Work out the finished part from the listing and answer in its coordinate system (mm). A direction names the side the tool comes from. Give positions to 0.01 mm unless a question says otherwise; leave off trailing zeros. Order: outer loops, then holes, each group sorted by start corner. A loop starts at its lowest first (then second) coordinate and runs counter-clockwise, first axis right, second up.
Autodesk Inventor part; units mm, degrees
ref_plane "YZ Plane" through (0, 0, 0) normal (1, 0, 0) x (0, 1, 0)
ref_plane "XZ Plane" through (0, 0, 0) normal (0, 1, 0) x (-1, 0, 0)
ref_plane "XY Plane" through (0, 0, 0) normal (0, 0, 1) x (1, 0, 0)
sketch "Sketch9" plane through (0, 0, 0) normal (0, 1, 0) x (-1, 0, 0)
  line L0 (-27, 35.5) -> (27, 35.5)
  line L1 (27, 35.5) -> (27, -35.5)
  line L2 (27, -35.5) -> (-27, -35.5)
  line L3 (-27, -35.5) -> (-27, 35.5)
  line L4 (-27, 35.5) -> (27, -35.5) construction
  line L5 (27, 35.5) -> (-27, -35.5) construction
  point P0 (0, 0)
  dimension "d39" = 54
  dimension "d40" = 71
extrude "Extrusion4" add sketch "Sketch9" along normal blind 10
sketch "Sketch10" plane through (0, 10, 0) normal (0, 1, 0) x (1, 0, 0)
  circle A0 centre (0, 0) radius 7.5
  dimension "d43" = 15
extrude "Extrusion5" cut sketch "Sketch10" against normal blind 10
sketch "Sketch11" plane through (27, 0, 35.5) normal (1, 0, 0) x (0, 0, -1)
  point P0 (35.5, 0)
  point P1 (35.5, 5)
hole "Hole5" at (27, 5, 0) direction (-1, 0, 0) diameter 3.242 depth 11.8 tip angle 118
sketch "Sketch12" plane through (0, 10, 0) normal (0, 1, 0) x (1, 0, 0)
  point P0 (0, 0)
sketch "Sketch13" plane through (0, 10, 0) normal (0, 1, 0) x (1, 0, 0)
  point P0 (0, 0)
  point P1 (22.809, -31.309)
  point P2 (-22.809, 31.309)
  point P3 (-22.809, -31.309)
  point P4 (22.809, 31.309)
hole "Hole6" at (-22.809, 10, 31.309) at (-22.809, 10, -31.309) at (22.809, 10, -31.309) at (22.809, 10, 31.309) direction (0, -1, 0) diameter 2.459 depth 8.8 tip angle 118
fillet "Fillet3" radius 4 4 edges at (-27, 5, -35.5) (-27, 5, 35.5) (27, 5, -35.5) (27, 5, 35.5)
sketch "Sketch14" plane through (23, 0, -35.5) normal (0, 0, -1) x (-1, 0, 0)
  point P0 (23, 0)
  point P1 (23, 5)
sketch "Sketch15" plane through (-23, 0, 35.5) normal (0, 0, 1) x (1, 0, 0)
  point P0 (23, 0)
  point P1 (23, 5)
hole "Hole7" at (0, 5, 35.5) direction (0, 0, -1) diameter 4 depth 20
hole "Hole8" at (0, 5, -35.5) direction (0, 0, 1) diameter 4 depth 20
sketch "Sketch16" plane through (0, 5, 15.5) normal (0, 0, 1) x (1, 0, 0)
  point P0 (0, -5)
  point P1 (0, 0)
sketch "Sketch17" plane through (0, 5, -15.5) normal (0, 0, -1) x (-1, 0, 0)
  point P0 (0, -5)
  point P1 (0, 0)
hole "Hole9" at (0, 5, -15.5) direction (0, 0, 1) diameter 3.242 depth 11.8
hole "Hole10" at (0, 5, 15.5) direction (0, 0, -1) diameter 3.242 depth 11.8
equation "\"z\" = 71"
equation "\"x\" = 54"
equation "\"corner\" = 4"
properties part number "CardMount_sjc"
1. The mould has two halves that part along X. Classify faces 1 (the face through (27, 3, 0)), 2 (the face through (-0.3, 2.7, -35.5)), 3 (the face through (1.2, 6.6, 25.4)): pulls with the +X half, pulls with the -X half, needs draft (parallel to the pull), parting line crosses it, or undercut.
Findings below:
face 1: pulls with the +X half
face 2: needs draft
face 3: undercut
2. The part is cut by section C-C (y = 8.5). Write down the section's boundary in (x, z), then the cut area to 3 significant figures.
Findings below:
outline: (-27, -31.5) arc R4 ccw to (-23, -35.5) - (23, -35.5) arc R4 ccw to (27, -31.5) - (27, 31.5) arc R4 ccw to (23, 35.5) - (-23, 35.5) arc R4 ccw to (-27, 31.5) - close; hole circle Ø2.46 at (-22.81, -31.31); hole circle Ø2.46 at (-22.81, 31.31); hole circle Ø15 at (0, 0); hole circle Ø2.46 at (22.81, -31.31); hole circle Ø2.46 at (22.81, 31.31)
area: 3,620 mm2
3. The part is cut by section B-B (z = -25.5). Write down the section's boundary in (x, y), then the cut area to 3 significant figures.
Findings below:
outline: (-27, 0) - (27, 0) - (27, 10) - (-27, 10) - close; hole circle Ø4 at (0, 5)
area: 527 mm2
4. The part is cut by section A-A (x = 0). Write down the section's boundary in (y, z).
Findings below:
outline: (0, -35.5) - (3, -35.5) - (3, -15.5) - (3.38, -15.5) - (3.38, -7.5) - (0, -7.5) - close; (0, 7.5) - (3.38, 7.5) - (3.38, 15.5) - (3, 15.5) - (3, 35.5) - (0, 35.5) - close; (6.62, -15.5) - (7, -15.5) - (7, -35.5) - (10, -35.5) - (10, -7.5) - (6.62, -7.5) - close; (6.62, 7.5) - (10, 7.5) - (10, 35.5) - (7, 35.5) - (7, 15.5) - (6.62, 15.5) - close
5. Straight lines are drawn through the part: probe 1 along X at (y, z) = (5, -11.25); probe 2 along Y at (x, z) = (0, -28); probe 3 along Y at (x, z) = (0, 13). For each, find the intervals that lie inside material, in ascending order.
Findings below:
probe 1: x = -27 to -1.62, 1.62 to 27
probe 2: y = 0 to 3, 7 to 10
probe 3: y = 0 to 3.38, 6.62 to 10
6. Given P1, Ø3.5, axis at x = 0, y = 5, coming from the -Z side, flat-ended and moving along its own axis, determine where the tip first touches the part or whether it passes through.
Findings below:
P1: stops at z = -15.5
7. Which of the six approach directions +Z, -Z, +X, -X, +Y, -Y give full straight-line access (tool end or side, diameter ignored) to faces 4 (the face through (0, 3, -25)), 5 (the face through (3.461, 5.07, 6.654)), 6 (the face through (23.557, 5.538, 30.333)), 7 (the face through (21.017, 6.438, -0.748))?
Findings below:
face 4: -Z
face 5: +Y, -Y
face 6: +Y
face 7: +X
